Geometry: see drawing. Coordinates: mm, zero at the bounding-box minimum. Coordinates: 2 decimals unless noted, no trailing zeros. Loops run counter-clockwise (first coordinate to the right, second up) from the corner with the lowest first, then second, coordinate; pieces in that order, holes last. Notation, with made-up numbers: (81.25, 6) -> (104.25, 6) arc R18 ccw to (104.25, 12) -> close; hole circle Ø1 at (84, 88). An arc over 180 degrees is marked (long way). One line per item, written item: value. Start each with the question number.
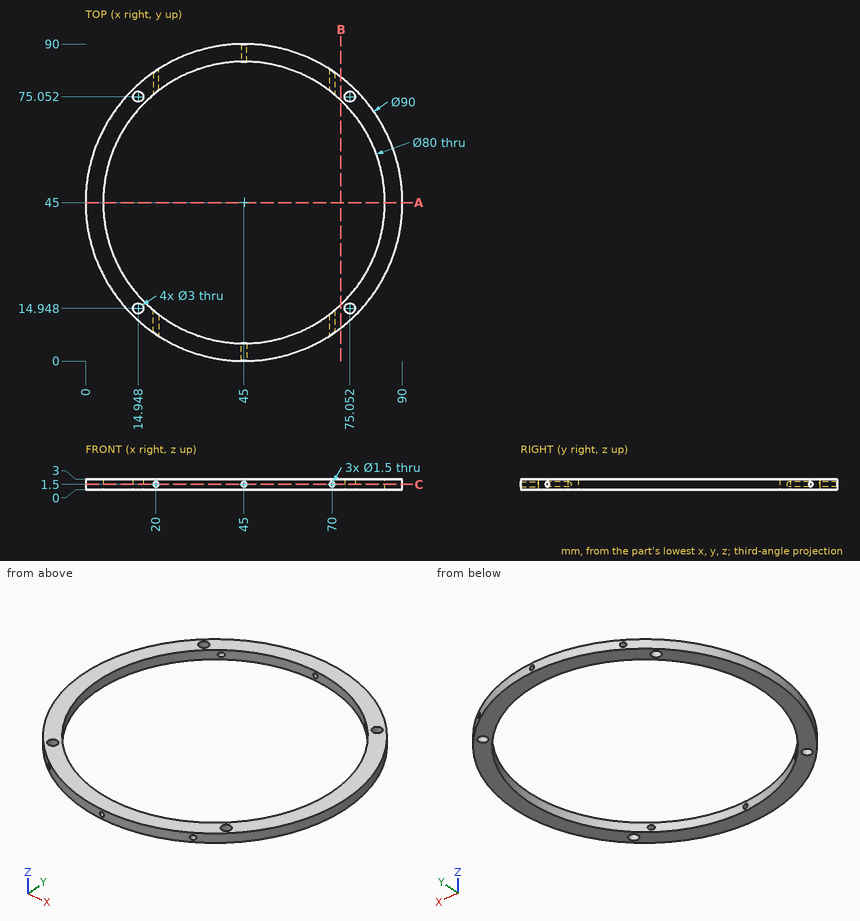
1. Pin query (flat end, axial travel): pin 1 Ø1 at (y, z) = (27, 0.5) entering from -X; pin 2 Ø1.2 at (x, z) = (45, 1.5) entering from +Y; pin 3 Ø1 at (x, z) = (42.5, 2) entering from -Y. Return the tip coordinate at first contact, or that it passes through.
2. Section C-C on z = 1.5. Count the separate pieces of the cut face and the enclosed holes in it, plus the area to 3 significant figures.
3. Section A-A on y = 45. Return the cut outline in (x, z), plus the area to 3 significant figures.
4. Section B-B on x = 72.5. Return the cut outline in (y, z).
5. Line query: L1, parallel to Z at x = 20, y = 79.75; L2, parallel to X at y = 79.5, z = 1.4; L3, parallel to Y at x = 14.5, z = 2.25. Output: solid intervals per line, ascending. Write a range as [from, to].
Checks:
1. pin 1: x = 3.54
1. pin 2: through
1. pin 3: y = 0.04
2. separate pieces: 6
2. enclosed holes: 4
2. area: 1,250 mm²
3. outline: (0, 0) -> (5, 0) -> (5, 3) -> (0, 3) -> close; (85, 0) -> (90, 0) -> (90, 3) -> (85, 3) -> close
3. area: 30.0 mm²
4. outline: (9.38, 0) -> (15.95, 0) -> (15.95, 3) -> (9.38, 3) -> close; (74.05, 0) -> (80.62, 0) -> (80.62, 3) -> (74.05, 3) -> close
5. L1: [0, 0.75], [2.25, 3]
5. L2: [16.11, 19.26], [20.74, 24.76], [65.24, 69.26], [70.74, 73.89]
5. L3: [11.91, 13.52], [16.38, 19.12], [70.88, 73.62], [76.48, 78.09]
